Part model, mm, in its own coordinate system. Face numbers are marked on the shaded views. Give positions to 0.01 mm unless a question says otherwise; leave off trailing zeros. Write each loop counter-clockwise with the first axis right and the second up, starting at its lowest first coordinate (ties: lowest second). Pieces come first, ordered by that corner, then holes.
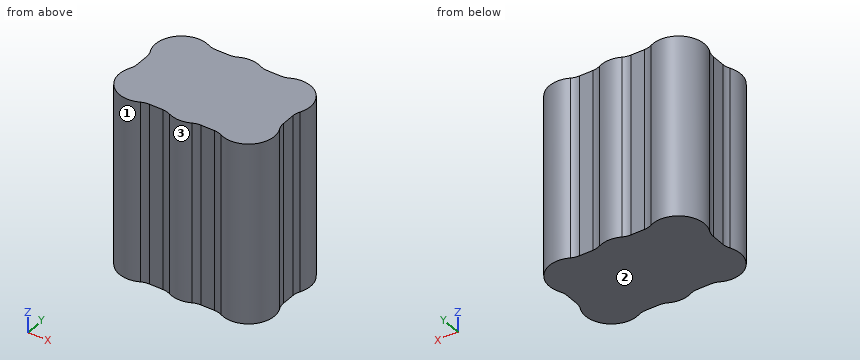
```python
from build123d import *

# Parameters (mm, degrees)
BOSS_EXTRUDE1_DEPTH = 64.6557


with BuildPart() as part:
    # Sketch1 → Boss-Extrude1 (new body)
    with BuildSketch(Plane.XY):
        with BuildLine():
            Line((3150.616152352, 2845.882200994), (3155.406404405, 2845.882200994))
            ThreePointArc((3155.406404405, 2845.882200994), (3156.838678555, 2845.718564285), (3158.197134553, 2845.236087848))
            ThreePointArc((3158.197134553, 2845.236087848), (3162.263228379, 2844.294700994), (3166.329322204, 2845.236087848))
            ThreePointArc((3166.329322204, 2845.236087848), (3167.687778202, 2845.718564285), (3169.120052352, 2845.882200994))
            Line((3169.120052352, 2845.882200994), (3173.910304405, 2845.882200994))
            ThreePointArc((3173.910304405, 2845.882200994), (3175.342578555, 2845.718564285), (3176.701034553, 2845.236087848))
            ThreePointArc((3176.701034553, 2845.236087848), (3187.309244963, 2847.00453441), (3189.077691525, 2857.61274482))
            ThreePointArc((3189.077691525, 2857.61274482), (3188.595215088, 2858.971200818), (3188.431578378, 2860.403474968))
            Line((3188.431578378, 2860.403474968), (3188.431578378, 2865.193727021))
            ThreePointArc((3188.431578378, 2865.193727021), (3188.595215088, 2866.626001171), (3189.077691525, 2867.984457169))
            ThreePointArc((3189.077691525, 2867.984457169), (3187.309244963, 2878.592667579), (3176.701034553, 2880.361114141))
            ThreePointArc((3176.701034553, 2880.361114141), (3175.342578555, 2879.878637704), (3173.910304405, 2879.715000994))
            Line((3173.910304405, 2879.715000994), (3169.120052352, 2879.715000994))
            ThreePointArc((3169.120052352, 2879.715000994), (3167.687778202, 2879.878637704), (3166.329322204, 2880.361114141))
            ThreePointArc((3166.329322204, 2880.361114141), (3162.263228379, 2881.302500994), (3158.197134553, 2880.361114141))
            ThreePointArc((3158.197134553, 2880.361114141), (3156.838678555, 2879.878637704), (3155.406404405, 2879.715000994))
            Line((3155.406404405, 2879.715000994), (3150.616152352, 2879.715000994))
            ThreePointArc((3150.616152352, 2879.715000994), (3149.183878202, 2879.878637704), (3147.825422204, 2880.361114141))
            ThreePointArc((3147.825422204, 2880.361114141), (3137.217211794, 2878.592667579), (3135.448765232, 2867.984457169))
            ThreePointArc((3135.448765232, 2867.984457169), (3135.931241669, 2866.626001171), (3136.094878379, 2865.193727021))
            Line((3136.094878379, 2865.193727021), (3136.094878379, 2860.403474968))
            ThreePointArc((3136.094878379, 2860.403474968), (3135.931241669, 2858.971200818), (3135.448765232, 2857.61274482))
            ThreePointArc((3135.448765232, 2857.61274482), (3137.217211794, 2847.00453441), (3147.825422204, 2845.236087848))
            ThreePointArc((3147.825422204, 2845.236087848), (3149.183878202, 2845.718564285), (3150.616152352, 2845.882200994))
        make_face()
    extrude(amount=BOSS_EXTRUDE1_DEPTH)


solid = part.part
```
1) Saw through at A-A, the plane z = 42. Write the cut outline in (x, y) (3 decimals).
Answers follow:
outline: (3135.449, 2857.613) arc R9.252 ccw to (3147.825, 2845.236) arc R6.35 cw to (3150.616, 2845.882) - (3155.406, 2845.882) arc R6.35 cw to (3158.197, 2845.236) arc R9.252 ccw to (3166.329, 2845.236) arc R6.35 cw to (3169.12, 2845.882) - (3173.91, 2845.882) arc R6.35 cw to (3176.701, 2845.236) arc R9.252 ccw to (3189.078, 2857.613) arc R6.35 cw to (3188.432, 2860.403) - (3188.432, 2865.194) arc R6.35 cw to (3189.078, 2867.984) arc R9.252 ccw to (3176.701, 2880.361) arc R6.35 cw to (3173.91, 2879.715) - (3169.12, 2879.715) arc R6.35 cw to (3166.329, 2880.361) arc R9.252 ccw to (3158.197, 2880.361) arc R6.35 cw to (3155.406, 2879.715) - (3150.616, 2879.715) arc R6.35 cw to (3147.825, 2880.361) arc R9.252 ccw to (3135.449, 2867.984) arc R6.35 cw to (3136.095, 2865.194) - (3136.095, 2860.403) arc R6.35 cw to start
2) Two-plate mould, pull along Y, no slides. Class the marked faces 1, 2 and 3: +Y half, -Y half, draft (parallel to the pull), parting line (faces both ways), or undercut.
Answers follow:
face 1: undercut
face 2: draft
face 3: -Y half
3) Wall check: L1, parallel to Y at x = 3153.5, z = 47.5 (3 decimals); L2, parallel to Y at x = 3162, z = 51.5; L3, parallel to X at y = 2862, z = 39.5. Give the ranges that are in metal, low to high.
Answers follow:
L1: y = 2845.882 to 2879.715
L2: y = 2844.3 to 2881.3
L3: x = 3136.09 to 3188.43
4) Saw through at C-C, the plane x = 3153.5. Write the cut outline in (y, z) (3 decimals).
Answers follow:
outline: (2845.882, 0) - (2879.715, 0) - (2879.715, 64.656) - (2845.882, 64.656) - close
5) Saw through at B-B, the plane y = 2863.5. Write the cut outline in (x, z).
Answers follow:
outline: (3136.09, 0) - (3188.43, 0) - (3188.43, 64.66) - (3136.09, 64.66) - close
6) Pin check, flat tips, straight feed: pin 1 Ø1.4 at (x, z) = (3154, 45.5) entering from +Y (3 decimals); pin 2 Ø5.5 at (x, z) = (3172.5, 45) entering from +Y; pin 3 Ø5 at (x, z) = (3170.5, 15) entering from +Y. Stop position of each tip, or through.
Answers follow:
pin 1: stops at y = 2879.715
pin 2: stops at y = 2879.86
pin 3: stops at y = 2879.81
